```python
from build123d import *

# Parameters (mm, degrees)
BOSS_EXTRUDE1_DEPTH                             = 5
CSK_FOR_M3_FLAT_HEAD_MACHINE_SCREW2_D           = 3.4
CSK_FOR_M3_FLAT_HEAD_MACHINE_SCREW2_CSINK_D     = 6.3
CSK_FOR_M3_FLAT_HEAD_MACHINE_SCREW2_CSINK_ANGLE = 90


with BuildPart() as part:
    # Sketch1 → Boss-Extrude1 (new body)
    with BuildSketch(Plane.XY):
        with BuildLine():
            Line((4.788497338, 51.358851364), (19.788497338, 1.438851364))
            ThreePointArc((19.788497338, 1.438851364), (19.012122681, -2.983768019), (15, -5))
            Line((15, -5), (-15, -5))
            ThreePointArc((-15, -5), (-19.012122681, -2.983768019), (-19.788497338, 1.438851364))
            Line((-19.788497338, 1.438851364), (-4.788497338, 51.358851364))
            ThreePointArc((-4.788497338, 51.358851364), (0, 54.92), (4.788497338, 51.358851364))
        make_face()
    extrude(amount=BOSS_EXTRUDE1_DEPTH)

    # CSK for M3 Flat Head Machine Screw2 (through all)
    with Locations(Plane(origin=(-15, 0, 0), x_dir=(-1, 0, 0), z_dir=(0, 0, -1))):
        with Locations((0, 0), (-15, 49.92), (-30, 0)):
            CounterSinkHole(CSK_FOR_M3_FLAT_HEAD_MACHINE_SCREW2_D / 2, CSK_FOR_M3_FLAT_HEAD_MACHINE_SCREW2_CSINK_D / 2, counter_sink_angle=CSK_FOR_M3_FLAT_HEAD_MACHINE_SCREW2_CSINK_ANGLE)


solid = part.part
```
Read the model definition and answer for the solid it produces. Units are mm, in the model's axes. Give positions to 0.01 mm unless a question says otherwise; leave off trailing zeros. Order: outer loops, then holes, each group sorted by start corner. A loop starts at its lowest first (then second) coordinate and runs counter-clockwise, first axis right, second up.
(1) Find section D-D (y = 49.92). Give the vertices of the cut face in (x, z), plus the area to 3 significant figures.
(2) Straight lines are drawn through the part: L1, parallel to X at y = 0, z = 3.6; L2, parallel to Y at x = 0, z = 2.3; L3, parallel to X at y = 1.5, z = 0.75. For each, find the intervals that lie inside material, in ascending order.
(3) Find section B-B (x = 0). Give the vertices of the cut face in (y, z).
(4) Find section A-A (y = 0). Give the vertices of the cut face in (x, z).
(5) Find section C-C (z = 2.8). Give the vertices of the cut face in (x, y), plus the area to 3 significant figures.
(6) For a pull along Y with two mould halves and no side action, classify faces 1 (the flat face through (12.2, 26.7, 2.5)), 2 (the cylindrical face through (-19, -3, 2)), 3 (the cylindrical face through (-13.38, 0.51, 3.25)) as released by +Y, released by -Y, zero draft, split by the parting line, or undercut.
(7) Given pin 1 (3 mm diameter, centred on x = -15, y = 0, fed in from -Z); pin 2 (2 mm diameter, centred on y = 15.5, z = 3.5, fed in from -X); pin 3 (8 mm diameter, centred on x = 7, y = 5, fed in from -Z); pin 4 (4 mm diameter, centred on x = 0, y = 49.92, fed in from -Z), each flat-ended and moving along its own axis, determine where each tip first touches the part or whether it passes through.
Result sheet:
1. outline: (-5.22, 0) - (-3.15, 0) - (-1.7, 1.45) - (-1.7, 5) - (-5.22, 5) - close; (1.7, 1.45) - (3.15, 0) - (5.22, 0) - (5.22, 5) - (1.7, 5) - close
1. area: 33.1 mm2
2. L1: x = -20 to -16.7, -13.3 to 13.3, 16.7 to 20
2. L2: y = -5 to 48.22, 51.62 to 54.92
2. L3: x = -19.77 to -16.87, -13.13 to 13.13, 16.87 to 19.77
3. outline: (-5, 0) - (46.77, 0) - (48.22, 1.45) - (48.22, 5) - (-5, 5) - close; (51.62, 1.45) - (53.07, 0) - (54.92, 0) - (54.92, 5) - (51.62, 5) - close
4. outline: (-20, 0) - (-18.15, 0) - (-16.7, 1.45) - (-16.7, 5) - (-20, 5) - close; (-13.3, 1.45) - (-11.85, 0) - (11.85, 0) - (13.3, 1.45) - (13.3, 5) - (-13.3, 5) - close; (16.7, 1.45) - (18.15, 0) - (20, 0) - (20, 5) - (16.7, 5) - close
5. outline: (-19.79, 1.44) arc R5 ccw to (-15, -5) - (15, -5) arc R5 ccw to (19.79, 1.44) - (4.79, 51.36) arc R5 ccw to (-4.79, 51.36) - close; hole circle Ø3.4 at (-15, 0); hole circle Ø3.4 at (0, 49.92); hole circle Ø3.4 at (15, 0)
5. area: 1,470 mm2
6. face 1: released by +Y
6. face 2: split by the parting line
6. face 3: undercut
7. pin 1: passes through
7. pin 2: stops at x = -15.86
7. pin 3: stops at z = 0
7. pin 4: stops at z = 1.15
